from build123d import *

# Parameters (mm, degrees)
EXTRUDE_THIN1_DEPTH = 76.2
EXTRUDE3_DEPTH      = 3.175


with BuildPart() as part:
    # Sketch1 → Extrude-Thin1 (new body)
    with BuildSketch(Plane(origin=(0, 0, 0), x_dir=(0, 0, -1), z_dir=(1, 0, 0))):
        with BuildLine():
            ThreePointArc((-40.374745946, 0), (12.536707256, 21.071210286), (65.448160458, 0))
            Line((65.448160458, 0), (63.702043982, -1.84463472))
            ThreePointArc((63.702043982, -1.84463472), (12.536707256, 18.531210286), (-38.628629469, -1.84463472))
            Line((-38.628629469, -1.84463472), (-40.374745946, 0))
        make_face()
    extrude(amount=-EXTRUDE_THIN1_DEPTH)

    # Sketch8 → Extrude3 (add, symmetric)
    with BuildSketch(Plane(origin=(-4.723115477, 0, 8.180675976), x_dir=(0.8660254037844382, 0, 0.500000000000001), z_dir=(-0.500000000000001, 0, 0.8660254037844382))):
        with BuildLine():
            Line((-26.019914049, 19.356414404), (-15.960161332, 62.469762483))
            ThreePointArc((-15.960161332, 62.469762483), (-15.889687792, 65.010575746), (-16.821324096, 67.375475819))
            ThreePointArc((-16.821324096, 67.375475819), (-36.428592093, 78.343903744), (-56.580491048, 68.411515413))
            ThreePointArc((-56.580491048, 68.411515413), (-57.544908965, 66.441876013), (-57.781782094, 64.261630063))
            Line((-57.781782094, 64.261630063), (-54.843835108, 19.356414404))
            Line((-54.843835108, 19.356414404), (-26.019914049, 19.356414404))
        make_face()
    extrude(amount=EXTRUDE3_DEPTH, both=True)


solid = part.part
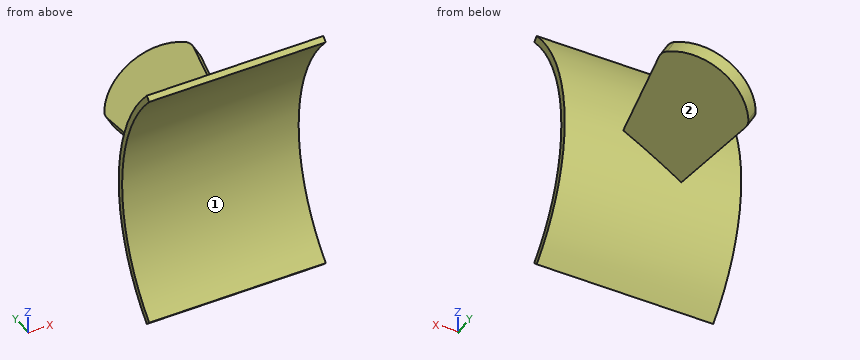
Work out the finished part from the listing and answer in its coordinate system (mm). Face numbers are marked on the shaded views. Round coordinates to 2 decimals unless told otherwise and drop trailing zeros. Loops run counter-clockwise (first coordinate to the right, second up) from the corner with the lowest first, then second, coordinate; pieces in that order, holes last. Notation, with made-up numbers: (89, 36.25) - (96, 36.25) arc R25 cw to (96, 57.25) - close; hole circle Ø6 at (-12.5, 12). An arc over 180 degrees is marked (long way). One line per item, written item: value.
Q1. Find section B-B on x = -15. Give the vertices of the cut face in (y, z), and give its area (3 significant figures).
Check values:
outline: (-1.84, -63.7) - (0, -65.45) arc R76.97 ccw to (0, 40.37) - (-1.84, 38.63) arc R74.43 cw to start
area: 291 mm2
Q2. Straight lines are drawn through the part: probe 1 along Z at (x, y) = (-9, 8); probe 2 along Y at (x, z) = (-22, -11.5); probe 3 along Z at (x, y) = (-65, 9). For each, find the intervals that lie inside material, in ascending order.
Check values:
probe 1: -55.45 to -50.7, 25.63 to 30.37
probe 2: 18.52 to 21.06
probe 3: -53.92 to -48.98, 23.9 to 28.85
Q3. Find section C-C on z = -32. Give the vertices of the cut face in (x, y).
Check values:
outline: (-76.2, 15.94) - (0, 15.94) - (0, 18.57) - (-76.2, 18.57) - close
Q4. Find section A-A on y = 11.5. Give the vertices of the cut face in (x, z), and give its area (3 significant figures).
Check values:
outline: (-76.2, -49.71) - (0, -49.71) - (0, -44.12) - (-76.2, -44.12) - close; (-76.2, 19.04) - (0, 19.04) - (0, 24.64) - (-76.2, 24.64) - close
area: 852 mm2
Q5. The mould has two halves that part along Y. Classify the marked faces 1 and 2: +Y half, -Y half, draft (parallel to the pull), parting line (faces both ways), or undercut.
Check values:
face 1: -Y half
face 2: draft
Q6. Each of these flat-tipped pins is pushed along its axis until it touches: pin 1 Ø1.5 at (x, z) = (-58, -44.5) entering from +Y; pin 2 Ø5 at (x, z) = (-8.5, -27) entering from +Y; pin 3 Ø8 at (x, z) = (-67.5, -22.5) entering from -Y. Where does it stop, or does it pass through?
Check values:
pin 1: y = 14.46
pin 2: y = 20.14
pin 3: y = 17.21
